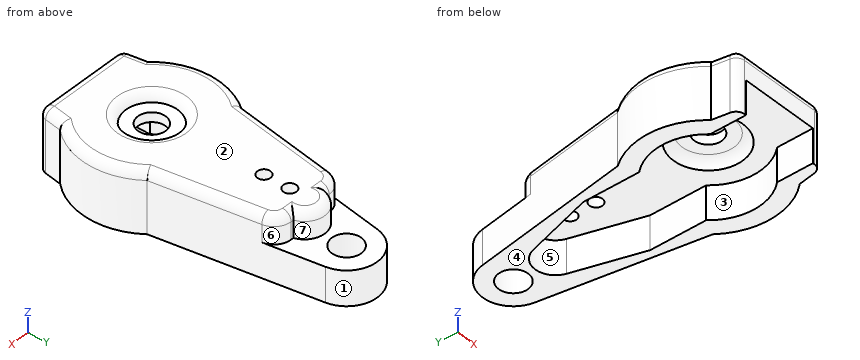
from build123d import *

# Parameters (mm, degrees)
SKETCH1_R                = 1.7
BOSS_EXTRUDE4_DEPTH      = 4
BOSS_EXTRUDE6_DEPTH      = 3
BOSS_EXTRUDE6_DEPTH_BACK = 0.1
SKETCH1_9_R              = 0.749999999999988
SKETCH1_9_R_2            = 0.749999999999991
SKETCH1_9_R_3            = 1.6
FILLET2_R                = 1
FILLET3_R                = 2
SKETCH2_R                = 4
CUT_EXTRUDE1_DEPTH       = 1
SKETCH3_R                = 3.0000000000000004
CUT_EXTRUDE2_DEPTH       = 1
FILLET4_R                = 1
FILLET5_R                = 1


# Some blends are built 0.0001 mm under size
with BuildPart() as part:
    # Sketch1 → Boss-Extrude4 (new body)
    with BuildSketch(Plane.XY):
        with BuildLine():
            Line((-3.5013415582545715, 23.136685369325342), (-6.388076465833109, 4.9802087372588275))
            ThreePointArc((-6.388076465833109, 4.9802087372588275), (-8.093690123038968, -0.31965636583910695), (-5.975409836065571, -5.468498632261951))
            Line((-5.9754098360655705, -5.468498632261951), (-5.531546482610164, -8.2602321522629))
            Line((-5.531546482610164, -8.2602321522629), (-4.5, -8.2602321522629))
            Line((-4.499999999999999, -8.2602321522629), (-4.500000000000003, -4.1182520563948))
            ThreePointArc((-4.500000000000003, -4.1182520563948), (-6.1, -6.7e-16), (-4.500000000000001, 4.118252056394799))
            Line((-4.5, 4.118252056394798), (-4.500000000000003, 10.602053391322137))
            Line((-4.500000000000003, 10.602053391322137), (-2.23677055895614, 18.353113855252126))
            ThreePointArc((-2.236770558956141, 18.353113855252126), (5.33e-15, 20.030171719280638), (2.2367705589561506, 18.353113855252126))
            Line((2.2367705589561497, 18.353113855252126), (4.499999999999999, 10.602053391322137))
            Line((4.499999999999999, 10.602053391322137), (4.500000000000003, 4.1182520563948))
            ThreePointArc((4.5000000000000036, 4.1182520563948), (6.099999999999998, -2.2e-16), (4.5, -4.118252056394798))
            Line((4.5, -4.118252056394798), (4.500000000000001, -8.260232152262898))
            Line((4.500000000000001, -8.2602321522629), (5.531546482610164, -8.2602321522629))
            Line((5.531546482610164, -8.2602321522629), (5.975409836065575, -5.468498632261945))
            ThreePointArc((5.975409836065576, -5.468498632261946), (8.093690123038972, -0.3196563658391036), (6.388076465833111, 4.9802087372588275))
            Line((6.388076465833109, 4.9802087372588275), (3.5013415582545715, 23.136685369325342))
            ThreePointArc((3.5013415582545715, 23.136685369325342), (-1.1e-16, 26.125319634106553), (-3.5013415582545715, 23.136685369325342))
        make_face()
        with Locations((0, 22.58)):
            Circle(SKETCH1_R, mode=Mode.SUBTRACT)
    extrude(amount=-BOSS_EXTRUDE4_DEPTH)

    # Sketch1<9> → Boss-Extrude6 (add, two sides: drawn at the far end of the back side and taken through both)
    with BuildSketch(Plane.XY.offset(-BOSS_EXTRUDE6_DEPTH_BACK)):
        with BuildLine():
            Line((-2.2367705589561404, 18.353113855252126), (-4.261891259190779, 18.353113855252126))
            Line((-4.261891259190779, 18.353113855252126), (-6.388076465833109, 4.9802087372588275))
            ThreePointArc((-6.388076465833109, 4.9802087372588275), (-8.093690123038968, -0.31965636583910695), (-5.975409836065571, -5.468498632261951))
            Line((-5.9754098360655705, -5.468498632261951), (-5.531546482610164, -8.2602321522629))
            Line((-5.531546482610164, -8.2602321522629), (5.531546482610164, -8.2602321522629))
            Line((5.531546482610164, -8.2602321522629), (5.975409836065575, -5.468498632261945))
            ThreePointArc((5.975409836065576, -5.468498632261946), (8.093690123038972, -0.3196563658391036), (6.388076465833111, 4.9802087372588275))
            Line((6.388076465833109, 4.9802087372588275), (4.261891259190779, 18.353113855252126))
            Line((4.261891259190779, 18.353113855252126), (2.2367705589561506, 18.353113855252126))
            ThreePointArc((2.2367705589561506, 18.353113855252126), (5.33e-15, 20.030171719280638), (-2.236770558956141, 18.353113855252126))
        make_face()
        with Locations((5.15e-15, 16)):
            Circle(SKETCH1_9_R, mode=Mode.SUBTRACT)
        with Locations((4.18e-15, 13.000000000000002)):
            Circle(SKETCH1_9_R_2, mode=Mode.SUBTRACT)
        Circle(SKETCH1_9_R_3, mode=Mode.SUBTRACT)
    extrude(amount=BOSS_EXTRUDE6_DEPTH + BOSS_EXTRUDE6_DEPTH_BACK)

    # Fillet2
    fillet2_edges = [part.edges().sort_by_distance(p)[0] for p in [
        (5.531546482610164, -8.2602321522629, -0.5),
        (-5.531546482610164, -8.2602321522629, -0.5),
        (0, -8.2602321522629, 3),
        (5.753478159337869, -6.864365392262423, 3),
        (-8.093690123038968, -0.3196563658391076, 3),
        (-5.324983862511944, 11.666661296255477, 3),
        (-3.2493309090734597, 18.353113855252126, 3),
        (3.249330909073465, 18.353113855252126, 3),
        (5e-15, 20.030171719280638, 3),
        (-5.753478159337868, -6.864365392262425, 3),
        (8.093690123038972, -0.31965636583910384, 3),
        (5.324983862511944, 11.666661296255477, 3),
    ]]
    fillet(fillet2_edges, radius=FILLET2_R)

    # Fillet3
    # the kernel refuses this fillet: 2 mm, written as the material it takes off along each edge
    with BuildSketch(Plane(origin=(-2.554754600251938, 16.35311385525213, 3), x_dir=(0, 1, 0), z_dir=(1, 0, 0))) as fillet3_piece_1:
        with BuildLine():
            CenterArc((1, -1), 1, 0, 90)
            Line((2, -1), (2, 0))
            Line((2, 0), (1, 0))
        make_face()
    revolve(axis=Axis((-2.554754600251938, 16.35311385525213, 3), (0, 0, 1)), revolution_arc=80.96604330855703, mode=Mode.SUBTRACT)
    with BuildSketch(Plane(origin=(2.554754600251939, 16.35311385525213, 3), x_dir=(0.9875954553070736, 0.15701979702194924, 0), z_dir=(0.15701979702194924, -0.9875954553070736, 0))) as fillet3_piece_2:
        with BuildLine():
            CenterArc((1, -1), 1, 0, 90)
            Line((2, -1), (2, 0))
            Line((2, 0), (1, 0))
        make_face()
    revolve(axis=Axis((2.554754600251939, 16.35311385525213, 3), (0, 0, 1)), revolution_arc=80.96604330855705, mode=Mode.SUBTRACT)
    with BuildSketch(Plane(origin=(4.261891259190781, 18.353113855252126, 3), x_dir=(0.15701979702194913, -0.9875954553070736, 0), z_dir=(0, 0, -1))) as fillet3_piece_3:
        with BuildLine():
            CenterArc((FILLET3_R * 0.853568329469, FILLET3_R), FILLET3_R, 189.03395669144297, 80.96604330855706)
            Line((-FILLET3_R * 0.134027125838, FILLET3_R * 0.842980202978), (0, 0))
            Line((0, 0), (FILLET3_R * 0.853568329469, -3e-17))
        make_face()
    extrude(amount=3, mode=Mode.SUBTRACT)
    with BuildSketch(Plane(origin=(-4.261891259190779, 18.353113855252126, 0), x_dir=(-0.15701979702194965, -0.9875954553070736, 0), z_dir=(0, 0, 1))) as fillet3_piece_4:
        with BuildLine():
            CenterArc((FILLET3_R * 0.853568329469, FILLET3_R), FILLET3_R, 189.033956691443, 80.96604330855706)
            Line((-FILLET3_R * 0.134027125838, FILLET3_R * 0.842980202978), (0, 0))
            Line((0, 0), (FILLET3_R * 0.853568329469, -3e-17))
        make_face()
    extrude(amount=3.000000000000001, mode=Mode.SUBTRACT)

    # Sketch2 → Cut-Extrude1 (cut)
    with BuildSketch(Plane(origin=(0, 0, -0.1), x_dir=(-1, 0, 0), z_dir=(0, 0, -1))):
        Circle(SKETCH2_R)
    extrude(amount=-CUT_EXTRUDE1_DEPTH, mode=Mode.SUBTRACT)

    # Sketch3 → Cut-Extrude2 (cut)
    with BuildSketch(Plane.XY.offset(3)):
        Circle(SKETCH3_R)
    extrude(amount=-CUT_EXTRUDE2_DEPTH, mode=Mode.SUBTRACT)

    # Fillet4
    fillet4_edges = [part.edges().sort_by_distance(p)[0] for p in [
        (4, 4.9e-16, 0.9),
    ]]
    fillet(fillet4_edges, radius=FILLET4_R - 0.0001)  # a hair under: the kernel refuses the full size

    # Fillet5
    fillet5_edges = [part.edges().sort_by_distance(p)[0] for p in [
        (-3.0000000000000004, 3.7e-16, 3),
    ]]
    fillet(fillet5_edges, radius=FILLET5_R - 0.0001)  # a hair under: the kernel refuses the full size


solid = part.part
Can you work these out from the model? Positions are in its coordinate system, mm. Face numbers are marked on the shaded views. A direction names the side the tool comes from. Coordinates: 2 decimals unless noted, no trailing zeros. Loops run counter-clockwise (first coordinate to the right, second up) from the corner with the lowest first, then second, coordinate; pieces in that order, holes last. Notation, with made-up numbers: M 22,-30 L 32,-30 A22 cw 32,-14 Z; hole C -31,33 d1. An arc over 180 degrees is marked long. Return JSON: item names as keys, results as strings. Group by question number.
Item 1: Thinking about a two-plate mould opening in X: for the marked faces 1, 2 and 3, which applies, released by +X, released by -X, zero draft, split by the parting line, or undercut?
Item 2: I'm going to push flat-ended pins straight in: pin 1 Ø3.5 at (x, y) = (-2, 4.5) entering from -Z; pin 2 Ø3 at (x, y) = (0, 0.5) entering from +Z; pin 3 Ø6.5 at (x, y) = (0, 0) entering from +Z; pin 4 Ø1.9 at (x, y) = (0, 0) entering from +Z. Where does each tip first touch, or does it pass through?
Item 3: Imagine slicing it at D-D (x = 0). Give the number of separate pieces and of enclosed holes in the cut face, and give its area (3 significant figures).
Item 4: If I drill on L1, parallel to X at y = 0, z = 2.05; L2, parallel to Z at x = -2.5, y = -6; L3, parallel to Z at x = -2.25, y = 1.5, over which ranges is the centre line in solid material (lowest first)? Write a range as from..to.
Item 5: On a 3-axis mill with a long thin cutter (end or side, diameter ignored), from which of +Z, -Z, +X, -X, +Y, -Y can I reach the whole of each face in a straight line? I mean the marked faces 4, 5, 6 and 7. Say none if no direction works.
Item 6: Imagine slicing it at B-B (z = -1.25). Please give me the cut outline in (x, y).
Item 7: Imagine slicing it at A-A (z = 1.25). Please give me the cut outline in (x, y).
Verdict:
{
 "1": {"face 1": "split by the parting line", "face 2": "zero draft", "face 3": "undercut"},
 "2": {"pin 1": "stops at z = -0.1", "pin 2": "stops at z = 2", "pin 3": "stops at z = 2.66", "pin 4": "passes through"},
 "3": {"separate pieces": "5", "enclosed holes": "0", "area": "71.2 mm^2"},
 "4": {"L1": "x = -8.1..-3, 3..8.1", "L2": "z = -0.1..3", "L3": "z = 0.9..2"},
 "5": {"face 4": "-Z, +X, -X, +Y, -Y", "face 5": "-Z, -Y", "face 6": "+Z, +X, +Y", "face 7": "+Z, +Y"},
 "6": {"outline": "M -6.39,4.98 A8.1 ccw -5.98,-5.47 L -5.67,-7.42 A1 ccw -4.68,-8.26 L -4.5,-8.26 L -4.5,-4.12 A6.1 cw -4.5,4.12 L -4.5,10.6 L -2.24,18.35 A2.33 cw 2.24,18.35 L 4.5,10.6 L 4.5,4.12 A6.1 cw 4.5,-4.12 L 4.5,-8.26 L 4.68,-8.26 A1 ccw 5.67,-7.42 L 5.98,-5.47 A8.1 ccw 6.39,4.98 L 3.5,23.14 A3.55 ccw -3.5,23.14 Z; hole C 0,22.58 d3.4"},
 "7": {"outline": "M -6.39,4.98 A8.1 ccw -5.98,-5.47 L -5.67,-7.42 A1 ccw -4.68,-8.26 L 4.68,-8.26 A1 ccw 5.67,-7.42 L 5.98,-5.47 A8.1 ccw 6.39,4.98 L 4.53,16.67 A2 ccw 2.55,18.35 L 2.24,18.35 A2.33 ccw -2.24,18.35 L -2.55,18.35 A2 ccw -4.53,16.67 Z; hole C 0,0 d3.2; hole C 0,13 d1.5; hole C 0,16 d1.5"}
}
